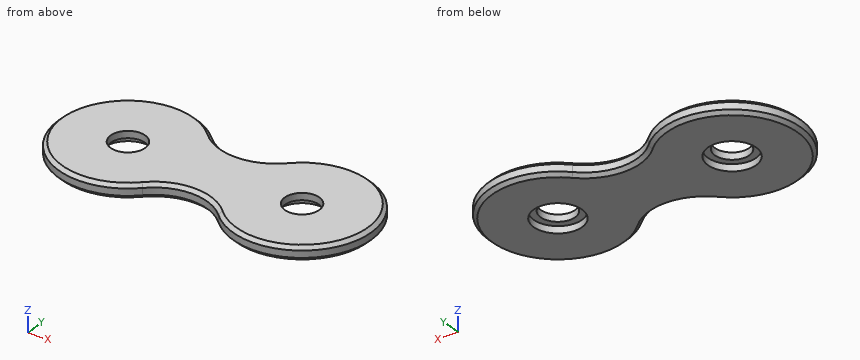
```python
from build123d import *

# Parameters (mm, degrees)
SKETCH1_R           = 2.5
BOSS_EXTRUDE1_DEPTH = 2
CHAMFER1_SIZE       = 0.5
SKETCH2_R           = 3.5
CUT_EXTRUDE1_DEPTH  = 1


with BuildPart() as part:
    # Sketch1 → Boss-Extrude1 (new body)
    with BuildSketch(Plane.XY):
        with BuildLine():
            ThreePointArc((17.928932188, -7.071067812), (35, 0), (17.928932188, 7.071067812))
            ThreePointArc((17.928932188, 7.071067812), (12.5, 4.82233047), (7.071067812, 7.071067812))
            ThreePointArc((7.071067812, 7.071067812), (-10, 0), (7.071067812, -7.071067812))
            ThreePointArc((7.071067812, -7.071067812), (12.5, -4.82233047), (17.928932188, -7.071067812))
        make_face()
        with Locations((25, 0)):
            Circle(SKETCH1_R, mode=Mode.SUBTRACT)
        Circle(SKETCH1_R, mode=Mode.SUBTRACT)
    extrude(amount=BOSS_EXTRUDE1_DEPTH)

    # Chamfer1
    chamfer1_edges = [part.edges().sort_by_distance(p)[0] for p in [
        (12.5, -4.82233047, 2),
        (35, 0, 2),
        (12.5, 4.82233047, 2),
        (35, 0, 0),
        (12.5, -4.82233047, 0),
        (-10, 0, 0),
        (12.5, 4.82233047, 0),
        (-10, 0, 2),
    ]]
    chamfer(chamfer1_edges, length=CHAMFER1_SIZE)

    # Sketch2 → Cut-Extrude1 (cut)
    with BuildSketch(Plane.XY):
        Circle(SKETCH2_R)
        with Locations((25, 0)):
            Circle(SKETCH2_R)
    extrude(amount=CUT_EXTRUDE1_DEPTH, mode=Mode.SUBTRACT)


solid = part.part
```
Geometry check sheet. Reference: the model listing, model coordinates, mm. Round coordinates to 2 decimals unless told otherwise and drop trailing zeros. Order: outer loops, then holes, each group sorted by start corner. A loop starts at its lowest first (then second) coordinate and runs counter-clockwise, first axis right, second up. Notation, with made-up numbers: (-20, 55.25) - (-4, 55.25) arc R15 ccw to (-4, 74.25) - close; hole circle Ø5 at (72, 74.5). An arc over 180 degrees is marked (long way). Use a Markdown table: item, result. Add a question column.
(1) Sectioned sample at B-B, the plane x = 0. Enter the section's corners in (y, z).
(2) Material ranges on line 1 along Y through (x, z) = (0, 0.65); line 2 along X through (y, z) = (-6, 1.95); line 3 along X through (y, z) = (-8.75, 1.85), recorded low to high. Write a range as [from, to].
(3) Sectioned sample at A-A, the plane y = 0. Enter the section's corners in (x, z).
Answers below:
| question | item | result |
|---|---|---|
| 1 | outline | (-10, 0.5) - (-9.5, 0) - (-3.5, 0) - (-3.5, 1) - (-2.5, 1) - (-2.5, 2) - (-9.5, 2) - (-10, 1.5) - close; (2.5, 1) - (3.5, 1) - (3.5, 0) - (9.5, 0) - (10, 0.5) - (10, 1.5) - (9.5, 2) - (2.5, 2) - close |
| 2 | line 1 | [-10, -3.5], [3.5, 10] |
| 2 | line 2 | [-7.43, 7.62], [17.38, 32.43] |
| 2 | line 3 | [-4.07, 4.07], [20.93, 29.07] |
| 3 | outline | (-10, 0.5) - (-9.5, 0) - (-3.5, 0) - (-3.5, 1) - (-2.5, 1) - (-2.5, 2) - (-9.5, 2) - (-10, 1.5) - close; (2.5, 1) - (3.5, 1) - (3.5, 0) - (21.5, 0) - (21.5, 1) - (22.5, 1) - (22.5, 2) - (2.5, 2) - close; (27.5, 1) - (28.5, 1) - (28.5, 0) - (34.5, 0) - (35, 0.5) - (35, 1.5) - (34.5, 2) - (27.5, 2) - close |
